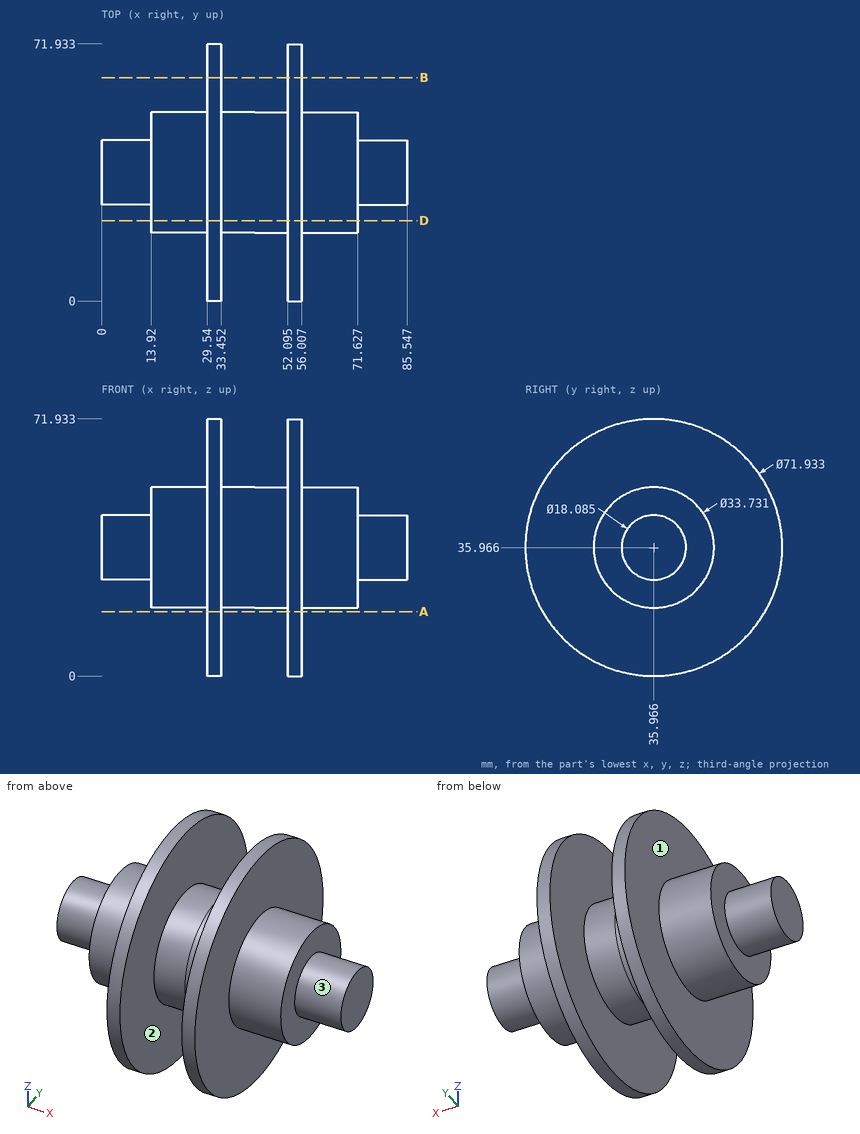
Here's the drawing with two shaded views (mm, measured from the low corner). I have some questions. A direction names the side the tool comes from. Give positions to 0.01 mm unless a question says otherwise; leave off trailing zeros. Write each loop counter-clockwise with the first axis right and the second up, starting at its lowest first coordinate (ties: lowest second). Pieces come first, ordered by that corner, then holes. Notation, with made-up numbers: (35, 37) - (42, 37) arc R7 cw to (42, 47) - close; hole circle Ø10 at (33.25, 74.5). An arc over 180 degrees is marked (long way). Write item = value, one per line. Start each with the question number.
1. Imagine slicing it at A-A (z = 18). Please give me the cut outline in (x, y) (1 decimal).
2. For pin 1 (6 mm diameter, centred on x = 62, z = 23.5, fed in from -Y); pin 2 (21.5 mm diameter, centred on y = 45, z = 54, fed in from -X); pin 3 (10 mm diameter, centred on y = 14, z = 35, fed in from -X), each with a flat end and sliding along its axis, tell me the tip position at first contact or that it passes through.
3. Imagine slicing it at D-D (y = 22.5). Please give me the cut outline in (x, z) (1 decimal), and give its area (4 significant figures).
4. Please list where these lines run through material, in increasing order: line 1 (X direction, y = 62, z = 23.5) (1 decimal); line 2 (X direction, y = 50.5, z = 28); line 3 (Y direction, x = 53, z = 69) (1 decimal).
5. Imagine slicing it at B-B (y = 62.5). Please give me the cut outline in (x, z) (1 decimal).
6. On a 3-axis mill with a long thin cutter (end or side, diameter ignored), from which of +Z, -Z, +X, -X, +Y, -Y can I reach the whole of each face in a straight line? I mean the marked faces 1, 2 and 3. Say none if no direction works.
Worked answers:
q1.outline = (29.5, 4.8) - (33.5, 4.8) - (33.5, 67.1) - (29.5, 67.1) - close; (52.1, 4.8) - (56, 4.8) - (56, 67.1) - (52.1, 67.1) - close
q2.pin_1 = 22.01
q2.pin_2 = 13.92
q2.pin_3 = 29.54
q3.outline = (13.9, 25.8) - (29.5, 25.8) - (29.5, 2.6) - (33.5, 2.6) - (33.5, 25.8) - (52.1, 25.8) - (52.1, 2.6) - (56, 2.6) - (56, 25.8) - (71.6, 25.8) - (71.6, 46.1) - (56, 46.1) - (56, 69.3) - (52.1, 69.3) - (52.1, 46.1) - (33.5, 46.1) - (33.5, 69.3) - (29.5, 69.3) - (29.5, 46.1) - (13.9, 46.1) - close
q3.area = 1,535 mm2
q4.line_1 = 29.5 to 33.5, 52.1 to 56
q4.line_2 = 13.92 to 71.63
q4.line_3 = 21.7 to 50.2
q5.outline = (29.5, 11.7) - (33.5, 11.7) - (33.5, 60.2) - (29.5, 60.2) - close; (52.1, 11.7) - (56, 11.7) - (56, 60.2) - (52.1, 60.2) - close
q6.face_1 = -X
q6.face_2 = none
q6.face_3 = +X
